Autodesk Inventor part; units mm, degrees
ref_plane "YZ Plane" through (0, 0, 0) normal (1, 0, 0) x (0, 1, 0)
ref_plane "XZ Plane" through (0, 0, 0) normal (0, 1, 0) x (-1, 0, 0)
ref_plane "XY Plane" through (0, 0, 0) normal (0, 0, 1) x (1, 0, 0)
sketch "Sketch1" plane through (0, 0, 0) normal (0, 1, 0) x (-1, 0, 0)
  line L0 (0, 0) -> (60.325, 0)
  line L1 (60.325, 0) -> (60.325, -9.525)
  line L2 (60.325, -9.525) -> (117.475, -9.525)
  line L3 (117.475, -9.525) -> (117.475, -104.775)
  line L4 (117.475, -104.775) -> (60.325, -104.775)
  line L5 (60.325, -104.775) -> (60.325, -114.3)
  line L6 (60.325, -114.3) -> (0, -114.3)
  line L7 (0, -114.3) -> (0, 0)
  dimension "d0" = 9.525
  dimension "d1" = 95.25
  dimension "d2" = 57.15
  dimension "d3" = 60.325
  dimension "d4" = 117.475
  dimension "d5" = 114.3
extrude "Extrusion1" add sketch "Sketch1" along normal blind 4.7625
sketch "Sketch2" plane through (0, 4.7625, 0) normal (0, 1, 0) x (1, 0, 0)
  line L0 (-117.475, 9.525) -> (-117.475, 104.775) construction
  line L1 (-117.475, 57.15) -> (0, 57.15) construction
  line L2 (-60.325, 0) -> (0, 0) construction
  line L3 (0, 0) -> (0, 114.3) construction
  line L4 (0, 114.3) -> (-60.325, 114.3) construction
  line L5 (-60.325, 114.3) -> (-60.325, 104.775) construction
  line L6 (-60.325, 104.775) -> (-117.475, 104.775) construction
  line L7 (-117.475, 104.775) -> (-117.475, 9.525) construction
  line L8 (-117.475, 9.525) -> (-60.325, 9.525) construction
  line L9 (-60.325, 9.525) -> (-60.325, 0) construction
  point P0 (-53.975, 4.7625)
  point P1 (-6.35, 4.7625)
  point P2 (-112.7125, 28.575)
  point P3 (-53.975, 109.5375)
  point P4 (-6.35, 109.5375)
  point P5 (-112.7125, 85.725)
  dimension "d8" = 6.35
  dimension "d9" = 6.35
  dimension "d10" = 4.7625
  dimension "d11" = 4.7625
  dimension "d12" = 19.05
  dimension "d13" = 4.7625
hole "Hole1" at (-53.975, 4.7625, -4.7625) at (-6.35, 4.7625, -4.7625) at (-112.7125, 4.7625, -28.575) at (-6.35, 4.7625, -109.5375) at (-53.975, 4.7625, -109.5375) at (-112.7125, 4.7625, -85.725) direction (0, -1, 0) diameter 4.4958 end through all countersink diameter 8.4328 countersink angle 82
sketch "Sketch3" plane through (0, 0, 0) normal (0, -1, 0) x (1, 0, 0)
  circle A0 centre (-53.975, -109.5375) radius 2.2479 construction
  circle A1 centre (-112.7125, -28.575) radius 2.2479 construction
  circle A2 centre (-53.975, -4.7625) radius 2.2479 construction
  circle A3 centre (-6.35, -4.7625) radius 2.2479 construction
  circle A4 centre (-6.35, -109.5375) radius 2.2479 construction
  circle A5 centre (-112.7125, -85.725) radius 2.2479 construction
  line L0 (0, 0) -> (-60.325, 0) construction
  line L1 (-60.325, 0) -> (-60.325, -9.525) construction
  line L2 (-60.325, -9.525) -> (-117.475, -9.525) construction
  line L3 (-117.475, -9.525) -> (-117.475, -104.775) construction
  line L4 (-117.475, -104.775) -> (-60.325, -104.775) construction
  line L5 (-60.325, -104.775) -> (-60.325, -114.3) construction
  line L6 (-60.325, -114.3) -> (0, -114.3) construction
  line L7 (0, -114.3) -> (0, 0) construction
  line L8 (0, -57.15) -> (-117.475, -57.15) construction
  point P0 (-88.9, -48.5775)
  point P1 (-107.95, -48.5775)
  point P2 (-88.9, -65.7225)
  point P3 (-107.95, -65.7225)
  dimension "d22" = 19.05
  dimension "d23" = 8.5725
  dimension "d24" = 8.5725
  dimension "d32" = 9.525
hole "Hole2" at (-88.9, 0, -48.5775) at (-107.95, 0, -48.5775) at (-88.9, 0, -65.7225) at (-107.95, 0, -65.7225) direction (0, 1, 0) diameter 4.4958 end through all countersink diameter 8.4328 countersink angle 82
sketch "Sketch4" plane through (0, 4.7625, 0) normal (0, 1, 0) x (1, 0, 0)
  line L0 (-47.625, 44.45) -> (-53.975, 44.45)
  line L1 (-57.15, 47.625) -> (-57.15, 66.675)
  line L2 (-53.975, 69.85) -> (-47.625, 69.85)
  line L3 (-44.45, 66.675) -> (-44.45, 47.625)
  line L4 (-44.45, 44.45) -> (-57.15, 69.85) construction
  line L5 (-57.15, 44.45) -> (-44.45, 69.85) construction
  line L6 (0, 0) -> (0, 114.3)
  line L7 (0, 57.15) -> (-50.8, 57.15) construction
  arc A0 (-53.975, 69.85) -> (-57.15, 66.675) centre (-53.975, 66.675) ccw
  arc A1 (-44.45, 66.675) -> (-47.625, 69.85) centre (-47.625, 66.675) ccw
  arc A2 (-47.625, 44.45) -> (-44.45, 47.625) centre (-47.625, 47.625) ccw
  arc A3 (-57.15, 47.625) -> (-53.975, 44.45) centre (-53.975, 47.625) ccw
  dimension "d33" = 50.8
  dimension "d34" = 12.7
  dimension "d35" = 25.4
  dimension "d36" = 3.175
extrude "Extrusion2" cut sketch "Sketch4" against normal through all
properties part number "ImagineFrameTopBot" material "SAN Plastic"
Design review of the part built by this model. Coordinates are the model's own, in mm. A direction names the side the tool comes from. Give positions to 0.01 mm unless a question says otherwise; leave off trailing zeros. Order: outer loops, then holes, each group sorted by start corner. A loop starts at its lowest first (then second) coordinate and runs counter-clockwise, first axis right, second up. Notation, with made-up numbers: (-34, 48.5) - (-27, 48.5) arc R36 cw to (-27, 83.5) - close; hole circle Ø5 at (-9, -39.75). An arc over 180 degrees is marked (long way). Write item = value, one per line. Start each with the question number.
Q1. Clearance check with flat-ended pins moving along their axes: pin 1 Ø5 at (x, z) = (-112.71, -28.58) entering from -Y; pin 2 Ø3.5 at (x, z) = (-6.35, -109.54) entering from +Y; pin 3 Ø1.4 at (x, y) = (-82.5, 3.5) entering from +Z (3 decimals); pin 4 Ø1.4 at (y, z) = (3, -3) entering from -X (3 decimals). State where each tip first meets the part, or that it passes through.
Q2. We need section B-B on x = -6.35. State the section outline as (y, z) points, plus the area to 3 significant figures.
Q3. To check wall thickness, follow L1, parallel to Z at x = -88.9, y = 3.8 (3 decimals); L2, parallel to X at y = 1.25, z = -60 (3 decimals); L3, parallel to X at y = 1.8, z = -4.5 (3 decimals). State the ranges of each line that lie inside material, in increasing order. Write a range as from..to.
Q4. We need section C-C on x = -88.9. State the section outline as (y, z) points (1 decimal).
Q5. Tool access review of faces 1 (the face through (-91.215, 2.123, -65.209)), 2 (the face through (-51, 2, -44.45)), 3 (the face through (-60.325, 2, -109)): name each direction out of +Z, -Z, +X, -X, +Y, -Y from which nothing blocks a thin tool from reaching the whole face with its end or side.
Q6. We need section D-D on y = 1.35. State how many separate pieces and enclosed holes the cut face has, plus the area to 3 significant figures.
Q7. Mouldability with a two-part tool opening along X and no side actions: class faces 4 (the face through (0, 2, -58)), 5 (the face through (-5.638, 2.64, -107.276)), 6 (the face through (-58, 4.762, -56)) as released by +X, released by -X, zero draft, split by the parting line, or undercut.
Working result:
q1.pin_1 = 0
q1.pin_2 = through
q1.pin_3 = -9.525
q1.pin_4 = -60.325
q2.outline = (0, -114.3) - (4.76, -114.3) - (4.76, -113.75) - (2.5, -111.79) - (0, -111.79) - close; (0, -107.29) - (2.5, -107.29) - (4.76, -105.32) - (4.76, -8.98) - (2.5, -7.01) - (0, -7.01) - close; (0, -2.51) - (2.5, -2.51) - (4.76, -0.55) - (4.76, 0) - (0, 0) - close
q2.area = 493 mm²
q3.L1 = -104.775..-67.97, -63.475..-50.825, -46.33..-9.525
q3.L2 = -117.475..-57.15, -44.45..0
q3.L3 = -60.325..-56.208, -51.742..-8.583, -4.117..0
q4.outline = (0, -104.8) - (4.8, -104.8) - (4.8, -68) - (2.3, -68) - (0, -69.9) - close; (0, -61.5) - (2.3, -63.5) - (4.8, -63.5) - (4.8, -50.8) - (2.3, -50.8) - (0, -52.8) - close; (0, -44.4) - (2.3, -46.3) - (4.8, -46.3) - (4.8, -9.5) - (0, -9.5) - close
q5.face_1 = -Y
q5.face_2 = +Y, -Y
q5.face_3 = -Z, -X, +Y, -Y
q6.separate_pieces = 1
q6.enclosed_holes = 11
q6.area = 11,800 mm²
q7.face_4 = released by +X
q7.face_5 = undercut
q7.face_6 = zero draft
